Read the model definition and answer for the solid it produces. Units are mm, in the model's axes. Face numbers are marked on the shaded views. A direction names the side the tool comes from. Coordinates: 2 decimals unless noted, no trailing zeros. Write each loop counter-clockwise with the first axis right and the second up, starting at its lowest first coordinate (ties: lowest second). Pieces come first, ordered by that corner, then holes. Notation, with made-up numbers: (72, -36.75) -> (112, -36.75) arc R9 ccw to (112, -21.75) -> close; hole circle Ø2 at (27, 7). An arc over 180 degrees is marked (long way). Use CSV: the item, a comma, the result in double quotes.
from build123d import *

# Parameters (mm, degrees)
SKETCH2_R           = 145
SKETCH2_R_2         = 105
SKETCH5_W           = 360
SKETCH5_H           = 360
SKETCH5_R           = 145
BOSS_EXTRUDE2_DEPTH = 50
SKETCH6_R           = 145
BOSS_EXTRUDE4_DEPTH = 50
SKETCH12_R          = 30
CUT_EXTRUDE2_DEPTH  = 10
SKETCH13_R          = 15
CUT_EXTRUDE4_DEPTH  = 40
CIRPATTERN3_COUNT   = 4
SKETCH14_R          = 30
CUT_EXTRUDE5_DEPTH  = 10
CUT_EXTRUDE6_START  = -50
SKETCH15_R          = 15
CUT_EXTRUDE6_DEPTH  = 40
CIRPATTERN4_COUNT   = 4


with BuildPart() as part:
    # Sweep-Thin2: sweep along a path in Sketch1
    with BuildLine(Plane.XY) as sweep_thin2_path:
        Line((0, 0), (-150, 0))
        ThreePointArc((-150, 0), (-296.448608391, 60.660999786), (-357.109608177, 207.109608177))
        Line((-357.109608177, 207.109608177), (-357.109608177, 357.109608177))
    # Sketch2 → Sweep-Thin2 (sweep)
    with BuildSketch(Plane(origin=(0, 0, 0), x_dir=(0, 0, -1), z_dir=(1, 0, 0))):
        Circle(SKETCH2_R)
        Circle(SKETCH2_R_2, mode=Mode.SUBTRACT)
    sweep(path=sweep_thin2_path.line)

    # Sketch5 → Boss-Extrude2 (add)
    with BuildSketch(Plane(origin=(0, 0, 0), x_dir=(0, 0, -1), z_dir=(1, 0, 0))):
        Rectangle(SKETCH5_W, SKETCH5_H)
        Circle(SKETCH5_R, mode=Mode.SUBTRACT)
    extrude(amount=-BOSS_EXTRUDE2_DEPTH)

    # Sketch6 → Boss-Extrude4 (add)
    with BuildSketch(Plane(origin=(0, 357.109608177, 0), x_dir=(1, 0, 0), z_dir=(0, 1, 0))):
        with BuildLine():
            Line((-537.109608177, 200), (-177.109608177, 200))
            ThreePointArc((-177.109608177, 200), (-162.967472553, 194.142135624), (-157.109608177, 180))
            Line((-157.109608177, 180), (-157.109608177, -180))
            ThreePointArc((-157.109608177, -180), (-162.967472553, -194.142135624), (-177.109608177, -200))
            Line((-177.109608177, -200), (-537.109608177, -200))
            ThreePointArc((-537.109608177, -200), (-551.2517438, -194.142135624), (-557.109608177, -180))
            Line((-557.109608177, -180), (-557.109608177, 180))
            ThreePointArc((-557.109608177, 180), (-551.2517438, 194.142135624), (-537.109608177, 200))
        make_face()
        with Locations((-357.109608177, 0)):
            Circle(SKETCH6_R, mode=Mode.SUBTRACT)
    extrude(amount=-BOSS_EXTRUDE4_DEPTH)

    # Sketch12 → Cut-Extrude2 (cut)
    with BuildSketch(Plane(origin=(0, 357.109608177, 0), x_dir=(1, 0, 0), z_dir=(0, 1, 0))):
        with Locations((-487.109608177, 130)):
            Circle(SKETCH12_R)
    cut_extrude2 = extrude(amount=-CUT_EXTRUDE2_DEPTH, mode=Mode.SUBTRACT)

    # Sketch13 → Cut-Extrude4 (cut)
    with BuildSketch(Plane(origin=(0, 347.109608177, 0), x_dir=(1, 0, 0), z_dir=(0, 1, 0))):
        with Locations((-487.109608177, 130)):
            Circle(SKETCH13_R)
    cut_extrude4 = extrude(amount=-CUT_EXTRUDE4_DEPTH, mode=Mode.SUBTRACT)

    # CirPattern3: Cut-Extrude2, Cut-Extrude4 ×4 about axis
    cirpattern3_axis = Axis((-357.109608177, 0, 0), (0, 1, 0))
    for i in range(1, CIRPATTERN3_COUNT):
        add(cut_extrude2.rotate(cirpattern3_axis, i * 360 / CIRPATTERN3_COUNT), mode=Mode.SUBTRACT)
        add(cut_extrude4.rotate(cirpattern3_axis, i * 360 / CIRPATTERN3_COUNT), mode=Mode.SUBTRACT)

    # Sketch14 → Cut-Extrude5 (cut)
    with BuildSketch(Plane(origin=(0, 0, 0), x_dir=(0, 0, -1), z_dir=(1, 0, 0))):
        with Locations((-130, 130)):
            Circle(SKETCH14_R)
    cut_extrude5 = extrude(amount=-CUT_EXTRUDE5_DEPTH, mode=Mode.SUBTRACT)

    # Sketch15 → Cut-Extrude6 (cut)
    with BuildSketch(Plane(origin=(0, 0, 0), x_dir=(0, 0, -1), z_dir=(1, 0, 0)).offset(CUT_EXTRUDE6_START)):
        with Locations((-130, 130)):
            Circle(SKETCH15_R)
    cut_extrude6 = extrude(amount=CUT_EXTRUDE6_DEPTH, mode=Mode.SUBTRACT)

    # CirPattern4: Cut-Extrude5, Cut-Extrude6 ×4 about axis
    cirpattern4_axis = Axis((0, 0, 0), (1, 0, 0))
    for i in range(1, CIRPATTERN4_COUNT):
        add(cut_extrude5.rotate(cirpattern4_axis, i * 360 / CIRPATTERN4_COUNT), mode=Mode.SUBTRACT)
        add(cut_extrude6.rotate(cirpattern4_axis, i * 360 / CIRPATTERN4_COUNT), mode=Mode.SUBTRACT)


solid = part.part
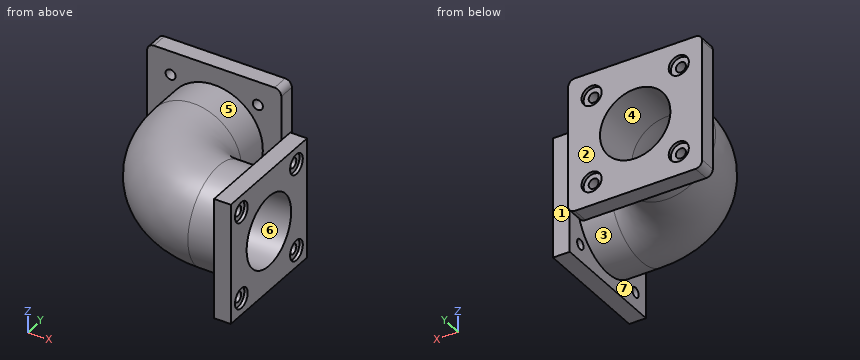
1. A cutting plane is placed at A-A (z = 0). Give the vertices of the cut face in (x, y).
Solutions:
outline,"(-557.11, 307.11) -> (-502.11, 307.11) -> (-502.11, 207.11) arc R352.11 ccw to (-150, -145) -> (-50, -145) -> (-50, -180) -> (0, -180) -> (0, -105) -> (-150, -105) arc R312.11 cw to (-462.11, 207.11) -> (-462.11, 357.11) -> (-557.11, 357.11) -> close; (-252.11, 207.11) arc R102.11 ccw to (-150, 105) -> (0, 105) -> (0, 180) -> (-50, 180) -> (-50, 145) -> (-150, 145) arc R62.11 cw to (-212.11, 207.11) -> (-212.11, 307.11) -> (-157.11, 307.11) -> (-157.11, 357.11) -> (-252.11, 357.11) -> close"
2. For a pull along Z with two mould halves and no side action, classify the marked faces 4, 5, 6 and 7 as pulls with the +Z half, pulls with the -Z half, needs draft (parallel to the pull), parting line crosses it, or undercut.
Solutions:
face 4,"undercut"
face 5,"parting line crosses it"
face 6,"undercut"
face 7,"needs draft"
3. A cutting plane is placed at C-C (y = 130). Give the number of separate pieces and of enclosed holes in the cut face, and give its area (3 significant figures).
Solutions:
separate pieces,"3"
enclosed holes,"1"
area,"66,500 mm^2"
4. Each of these flat-tipped pins is pushed along its axis until it touches: pin 1 Ø24 at (y, z) = (130, -130) entering from -X; pin 2 Ø4 at (x, z) = (-145, 28) entering from +Y; pin 3 Ø3 at (x, z) = (-484, -109) entering from +Y. Where does it stop, or does it pass through?
Solutions:
pin 1,"stops at x = -431.29"
pin 2,"stops at y = 142.65"
pin 3,"stops at y = 347.11"
5. A tool of negligible diameter and unlimited length cuts with its end or side. For the marked faces 1, 2 and 3, from which of +Z, -Z, +X, -X, +Y, -Y can it reach the whole face along a straight path? Write none if from no direction.
Solutions:
face 1,"+Z, -Z, +X, +Y"
face 2,"+Z, -Z, +X, -X, +Y"
face 3,"none"
6. A cutting plane is placed at B-B (x = -75.5). Give the vertices of the cut face in (y, z).
Solutions:
outline,"circle Ø290 at (0, 0); hole circle Ø210 at (0, 0)"
7. Find the intervals of material crossed by line 1 along Z through (x, y) = (-22, -130); line 2 along Z through (x, y) = (-363, 259); line 3 along Y through (x, z) = (-176, 84), in increasing order.
Solutions:
line 1,"z = -180 to -145, -115 to 115, 145 to 180"
line 2,"z = -144.88 to -104.83, 104.83 to 144.88"
line 3,"y = -117.15 to -61.75, 65.36 to 122.08, 307.11 to 357.11"
